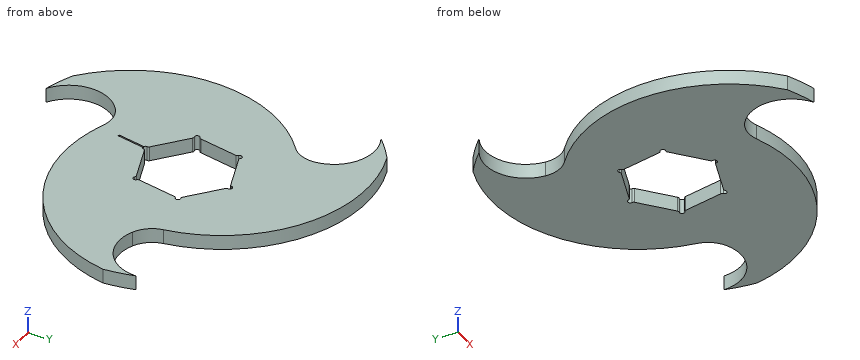
```python
from build123d import *

# Parameters (mm, degrees)
BOSS_EXTRUDE1_DEPTH = 2.5
FILLET1_R           = 10
CUT_EXTRUDE1_DEPTH  = 0.5


with BuildPart() as part:
    # Sketch1 → Boss-Extrude1 (new, symmetric)
    with BuildSketch(Plane.XY):
        with BuildLine():
            ThreePointArc((-42.426406871, 42.426406871), (-26.29235792, 40.654943242), (-22.609103215, 24.847373735))
            ThreePointArc((-22.609103215, 24.847373735), (-43.353983992, -14.099744614), (-25.343982725, -54.38457998))
            ThreePointArc((-25.343982725, -54.38457998), (-20.514410827, -56.38403097), (-15.529142706, -57.955549577))
            ThreePointArc((-15.529142706, -57.955549577), (-22.062034677, -43.097321505), (-10.213905264, -32.003744609))
            ThreePointArc((-10.213905264, -32.003744609), (33.887729018, -30.495779185), (59.7704192, 5.243757117))
            ThreePointArc((59.7704192, 5.243757117), (59.087208601, 10.426014565), (57.955549577, 15.529142706))
            ThreePointArc((57.955549577, 15.529142706), (48.354392597, 2.442378263), (32.82300848, 7.156370874))
            ThreePointArc((32.82300848, 7.156370874), (9.466254973, 44.595523799), (-34.426436475, 49.140822863))
            ThreePointArc((-34.426436475, 49.140822863), (-38.572797774, 45.958016405), (-42.426406871, 42.426406871))
        make_face()
        with BuildLine():
            Line((1.521012626, 15.824554357), (-11.336990739, 11.14462386))
            ThreePointArc((-11.336990739, 11.14462386), (-11.76671434, 11.107027916), (-12.157663867, 11.289330674))
            ThreePointArc((-12.157663867, 11.289330674), (-13.331690578, 11.186616647), (-13.22897655, 10.012589936))
            ThreePointArc((-13.22897655, 10.012589936), (-12.981555707, 9.659236353), (-12.943959764, 9.229512752))
            Line((-12.943959764, 9.229512752), (-15.320022748, -4.245810053))
            ThreePointArc((-15.320022748, -4.245810053), (-15.502325506, -4.63675958), (-15.855679089, -4.884180422))
            ThreePointArc((-15.855679089, -4.884180422), (-16.353739487, -5.952274392), (-15.285645517, -6.45033479))
            ThreePointArc((-15.285645517, -6.45033479), (-14.855921916, -6.412738847), (-14.46497239, -6.595041605))
            Line((-14.46497239, -6.595041605), (-3.983032008, -15.390433913))
            ThreePointArc((-3.983032008, -15.390433913), (-3.735611166, -15.743787496), (-3.698015222, -16.173511097))
            ThreePointArc((-3.698015222, -16.173511097), (-3.02204891, -17.138891039), (-2.056668967, -16.462924726))
            ThreePointArc((-2.056668967, -16.462924726), (-1.874366209, -16.071975199), (-1.521012626, -15.824554357))
            Line((-1.521012626, -15.824554357), (11.336990739, -11.14462386))
            ThreePointArc((11.336990739, -11.14462386), (11.76671434, -11.107027916), (12.157663867, -11.289330674))
            ThreePointArc((12.157663867, -11.289330674), (13.331690578, -11.186616647), (13.22897655, -10.012589936))
            ThreePointArc((13.22897655, -10.012589936), (12.981555707, -9.659236353), (12.943959764, -9.229512752))
            Line((12.943959764, -9.229512752), (15.320022748, 4.245810053))
            ThreePointArc((15.320022748, 4.245810053), (15.502325506, 4.63675958), (15.855679089, 4.884180422))
            ThreePointArc((15.855679089, 4.884180422), (16.353739487, 5.952274392), (15.285645517, 6.45033479))
            ThreePointArc((15.285645517, 6.45033479), (14.855921916, 6.412738847), (14.46497239, 6.595041605))
            Line((14.46497239, 6.595041605), (3.983032008, 15.390433913))
            ThreePointArc((3.983032008, 15.390433913), (3.735611166, 15.743787496), (3.698015222, 16.173511097))
            ThreePointArc((3.698015222, 16.173511097), (3.02204891, 17.138891039), (2.056668967, 16.462924726))
            ThreePointArc((2.056668967, 16.462924726), (1.874366209, 16.071975199), (1.521012626, 15.824554357))
        make_face(mode=Mode.SUBTRACT)
    extrude(amount=BOSS_EXTRUDE1_DEPTH, both=True)

    # Fillet1
    fillet1_edges = [part.edges().sort_by_distance(p)[0] for p in [
        (32.82300848, 7.156370874, 0),
        (-10.213905264, -32.003744609, 0),
        (-22.609103215, 24.847373735, 0),
    ]]
    fillet(fillet1_edges, radius=FILLET1_R)

    # Sketch2 → Cut-Extrude1 (cut)
    with BuildSketch(Plane.XY.offset(2.5)):
        Polygon((-3.181426759, -16.603075118), (-2.689022882, -16.689899207), (-4.425504659, -26.537976737), (-4.917908536, -26.451152648), align=None)
    extrude(amount=-CUT_EXTRUDE1_DEPTH, mode=Mode.SUBTRACT)


solid = part.part
```
The listing builds one solid part. Answer for the finished solid, in the listing's coordinates (mm). Round coordinates to 2 decimals unless told otherwise and drop trailing zeros. Order: outer loops, then holes, each group sorted by start corner. A loop starts at its lowest first (then second) coordinate and runs counter-clockwise, first axis right, second up. Notation, with made-up numbers: (-27.75, -14.5) - (-1.75, -14.5) arc R28 ccw to (-1.75, 14.5) - close; hole circle Ø6 at (-33, -39). An arc over 180 degrees is marked (long way). Put each result on its own line as item: value. Start each with the question number.
(1) Given P1, Ø2, axis at y = -29, z = -0.5, coming from the -X side; P2, Ø2, axis at y = 22.5, z = 0.5, coming from the -X side, each flat-ended and moving along its own axis, determine where each tip first touches the part or whether it passes through.
(2) Find section C-C (x = 27). Give the vertices of the cut face in (y, z), plus the area to 3 significant figures.
(3) Find section A-A (x = 6.5). Give the vertices of the cut face in (y, z).
(4) Find section D-D (x = -33). Give the vertices of the cut face in (y, z), plus the area to 3 significant figures.
(5) Find section B-B (y = -22.5). Give the vertices of the cut face in (x, z), plus the area to 3 significant figures.
(6) Straight lines are drawn through the part: probe 1 along Y at (x, z) = (-16, 0.6); probe 2 along Y at (x, z) = (-5, -2.2); probe 3 along Y at (x, z) = (-25.5, -1.35). For each, find the intervals that lie inside material, in ascending order. Write a range as from..to.
Reply:
1. P1: x = -41.89
1. P2: x = -26.75
2. outline: (-33.52, -2.5) - (25.97, -2.5) - (25.97, 2.5) - (-33.52, 2.5) - close
2. area: 297 mm^2
3. outline: (-36.24, -2.5) - (-12.91, -2.5) - (-12.91, 2.5) - (-36.24, 2.5) - close; (13.28, -2.5) - (46.31, -2.5) - (46.31, 2.5) - (13.28, 2.5) - close
4. outline: (-46.41, -2.5) - (14.75, -2.5) - (14.75, 2.5) - (-46.41, 2.5) - close; (43.95, -2.5) - (49.64, -2.5) - (49.64, 2.5) - (43.95, 2.5) - close
4. area: 334 mm^2
5. outline: (-42.94, -2.5) - (44.96, -2.5) - (44.96, 2.5) - (-3.71, 2.5) - (-3.71, 2) - (-4.22, 2) - (-4.22, 2.5) - (-42.94, 2.5) - close
5. area: 439 mm^2
6. probe 1: -57.83..-57.66, -34.17..-6.38, -4.95..52.2
6. probe 2: -34..-14.54, 13.45..50.73
6. probe 3: -54.25..22.59, 39.89..51.51
